Build history of the part. All positions in model axes, mm. A direction names the side the tool comes from. Round coordinates to 2 decimals unless told otherwise and drop trailing zeros. Order: outer loops, then holes, each group sorted by start corner. A loop starts at its lowest first (then second) coordinate and runs counter-clockwise, first axis right, second up. Notation, with made-up numbers: M 89,74.25 L 98,74.25 A10 cw 98,84.25 Z; hole C -40,11 d6. An arc over 180 degrees is marked long. One line per item, written item: value. Start each with the question number.
Item 1: Band-saw the part on A-A, the plane z = 77. Write the cut outline in (x, y), then the cut area to 3 significant figures.
Item 2: Pin check, flat tips, straight feed: pin 1 (12 mm diameter, centred on x = -86, y = -28.5, fed in from +Z); pin 2 (4 mm diameter, centred on y = -16, z = 41, fed in from +X); pin 3 (1.3 mm diameter, centred on y = -0.5, z = 243, fed in from +X) (3 decimals). Stop position of each tip, or through.
Item 3: Band-saw the part on B-B, the plane x = 91.5. Write the cut outline in (y, z), then the cut area to 3 significant figures.
Item 4: Band-saw the part on C-C, the plane z = 120.65. Write the cut outline in (x, y), then the cut area to 3 significant figures.
Item 5: Band-saw the part on D-D, the plane y = -41. Write the cut outline in (x, z).
Item 6: Probe L1, parallel to Z at x = 117, y = 6.5; L2, parallel to X at y = 36, z = 89; L3, parallel to Y at x = 0, z = 231 (3 decimals). List the from-to ranges inside material, lowest first.
Item 7: Two-plate mould, pull along X, no slides. Class faces 1 (the flat face through (-2, 16, 241.3)), 2 (the cylindrical face through (-96.2, 4.7, 9.4)), 3 (the flat face through (177.8, -1, 232)): +X half, -X half, draft (parallel to the pull), parting line (faces both ways), or undercut.
Item 8: Tool access for faces 4 (the flat face through (175, -74, 222.25)), 5 (the flat face through (-158.75, 16, 119)), 6 (the flat face through (114.3, 0, 232)): list every direction of +Z, -Z, +X, -X, +Y, -Y with a clear straight run to the whole face (end or side of a thin tool).
```python
from build123d import *

# Parameters (mm, degrees)
F0_W      = 355.6
F0_H      = 152.4
F1_DEPTH  = 19.05
F2_W      = 19.05
F2_H      = 152.4
F3_DEPTH  = 222.25
F5_DEPTH  = 184.15
F6_W      = 152.4
F6_H      = 19.05
F7_DEPTH  = 336.55
F5_FACE_R = 12.7
F8_DEPTH  = 25.4
F9_R      = 6.35
F10_DEPTH = 25.4
F13_DEPTH = 19.05
F14_R     = 3.175
F16_DEPTH = 19.05
F17_W     = 19.05
F17_H     = 19.05
F18_DEPTH = 3.81
F19_W     = 19.05
F19_H     = 19.05
F20_DEPTH = 2.54
F22_D     = 13.97


with BuildPart() as f1:
    # F0 (on Top) → F1 (new body)
    with BuildSketch(Plane.XY):
        Rectangle(F0_W, F0_H)
    extrude(amount=F1_DEPTH)

    # F2 (on face) → F3 (join)
    with BuildSketch(Plane.XY.offset(19.05)):
        with Locations((-168.275, 0)):
            Rectangle(F2_W, F2_H)
    extrude(amount=F3_DEPTH)

    # F4 (on face) → F5 (join)
    with BuildSketch(Plane.XY.offset(19.05)):
        with BuildLine():
            ThreePointArc((165.1, 76.2), (156.119744, 54.519744), (177.8, 63.5))
            ThreePointArc((177.8, 63.5), (174.080256, 72.480256), (165.1, 76.2))
        make_face()
        with BuildLine():
            ThreePointArc((165.1, -76.2), (174.080256, -72.480256), (177.8, -63.5))
            ThreePointArc((177.8, -63.5), (156.119744, -54.519744), (165.1, -76.2))
        make_face()
    extrude(amount=F5_DEPTH)

    # F6 (on face) → F7 (join)
    with BuildSketch(Plane.YZ.offset(-158.75)):
        with Locations((0, 231.775)):
            Rectangle(F6_W, F6_H)
    extrude(amount=F7_DEPTH)

    # F5_face (on face) → F8 (join)
    with BuildSketch(Plane(origin=(165.1, 63.5, 203.2), x_dir=(1, 0, 0), z_dir=(0, 0, 1))):
        Circle(F5_FACE_R)
        with Locations((0, -127)):
            Circle(F5_FACE_R)
    extrude(amount=F8_DEPTH)

    # F9 (on face) → F10 (cut)
    with BuildSketch(Plane(origin=(-177.8, 0, 0), x_dir=(0, -1, 0), z_dir=(-1, 0, 0))):
        with Locations((0, 120.65)):
            Circle(F9_R)
    extrude(amount=-F10_DEPTH, mode=Mode.SUBTRACT)

    # F12 (on face) → F13 (cut)
    with BuildSketch(Plane.XY.offset(241.3)):
        with BuildLine():
            Line((114.3, -25.4), (114.3, 25.4))
            ThreePointArc((114.3, 25.4), (107.95, 31.75), (101.6, 25.4))
            Line((101.6, 25.4), (101.6, -25.4))
            ThreePointArc((101.6, -25.4), (107.95, -31.75), (114.3, -25.4))
        make_face()
    extrude(amount=-F13_DEPTH, mode=Mode.SUBTRACT)

    # F14 (on face) → F16 (cut)
    with BuildSketch(Plane.XY.offset(241.3)):
        Circle(F14_R)
    extrude(amount=-F16_DEPTH, mode=Mode.SUBTRACT)

    # F17 (on face) → F18 (join)
    with BuildSketch(Plane.XY.offset(19.05)):
        with Locations((146.05, 0)):
            Rectangle(F17_W, F17_H)
    extrude(amount=F18_DEPTH)

    # F19 (on face) → F20 (join)
    with BuildSketch(Plane.XY.offset(241.3)):
        with Locations((146.05, 0)):
            Rectangle(F19_W, F19_H)
    extrude(amount=F20_DEPTH)

    # F22 (through all)
    with Locations(Plane.XY.offset(241.3)):
        with Locations((-101.365335, 0)):
            Hole(F22_D / 2)


solid = f1.part
```
Output:
1. outline: M -177.8,-76.2 L -158.75,-76.2 L -158.75,76.2 L -177.8,76.2 Z; C 165.1,-63.5 d25.4; C 165.1,63.5 d25.4
1. area: 3,920 mm²
2. pin 1: stops at z = 241.3
2. pin 2: stops at x = -158.75
2. pin 3: stops at x = 155.575
3. outline: M -76.2,0 L 76.2,0 L 76.2,19.05 L -76.2,19.05 Z; M -76.2,222.25 L 76.2,222.25 L 76.2,241.3 L -76.2,241.3 Z
3. area: 5,810 mm²
4. outline: M -177.8,-76.2 L -158.75,-76.2 L -158.75,-6.35 L -177.8,-6.35 Z; M -177.8,6.35 L -158.75,6.35 L -158.75,76.2 L -177.8,76.2 Z; C 165.1,-63.5 d25.4; C 165.1,63.5 d25.4
4. area: 3,670 mm²
5. outline: M -177.8,0 L 177.8,0 L 177.8,19.05 L -158.75,19.05 L -158.75,222.25 L 177.8,222.25 L 177.8,241.3 L -177.8,241.3 Z
6. L1: z = 0 to 19.05, 222.25 to 241.3
6. L2: x = -177.8 to -158.75
6. L3: y = -76.2 to -3.175, 3.175 to 76.2
7. face 1: draft
7. face 2: undercut
7. face 3: +X half
8. face 4: +X, -Y
8. face 5: +Y, -Y
8. face 6: +Z
